Could you check a few things on this model? Use its own coordinates, in mm. A direction names the side the tool comes from. Give positions to 0.01 mm unless a question says otherwise; leave off trailing zeros. Loops run counter-clockwise (first coordinate to the right, second up) from the corner with the lowest first, then second, coordinate; pieces in that order, holes last. Notation, with made-up numbers: (-3, 57) - (13, 57) arc R21 ccw to (13, 74) - close; hole circle Ø7 at (51, 69). An arc over 180 degrees is marked (long way). Use CSV: the item, a comma, the result in double quotes.
from build123d import *

# Parameters (mm, degrees)
ESQUISSE1_W             = 12
ESQUISSE1_H             = 108
ESQUISSE1_R             = 1.6
BOSS_EXTRU_1_DEPTH      = 4
ESQUISSE2_R             = 2.2
BOSS_EXTRU_2_DEPTH      = 4
BOSS_EXTRU_3_DEPTH      = 12
ESQUISSE4_W             = 12
ESQUISSE4_H             = 16
ESQUISSE4_R             = 2.2
BOSS_EXTRU_4_DEPTH      = 6
ENL_V_MAT_EXTRU_1_DEPTH = 13
ESQUISSE6_R             = 4.5
ENL_V_MAT_EXTRU_2_DEPTH = 14
ESQUISSE8_R             = 4.5
ENL_V_MAT_EXTRU_3_DEPTH = 4
ESQUISSE9_R             = 1.6
ENL_V_MAT_EXTRU_4_DEPTH = 17
ESQUISSE10_R            = 3.5
ENL_V_MAT_EXTRU_5_DEPTH = 14
CONG_1_R                = 4
CONG_2_R                = 4
CONG_3_R                = 4


with BuildPart() as part:
    # Esquisse1 → Boss.-Extru.1 (new body)
    with BuildSketch(Plane.XY):
        with Locations((-47.5, 54)):
            Rectangle(ESQUISSE1_W, ESQUISSE1_H)
        with Locations((-47.5, 100)):
            Circle(ESQUISSE1_R, mode=Mode.SUBTRACT)
    extrude(amount=BOSS_EXTRU_1_DEPTH)

    # Esquisse2 → Boss.-Extru.2 (add)
    with BuildSketch(Plane.XZ):
        Polygon((-41.5, 0), (-29.5, 0), (-29.5, 16), (-53.5, 16), (-53.5, 4), (-41.5, 4), align=None)
        with Locations((-37.5, 8)):
            Circle(ESQUISSE2_R, mode=Mode.SUBTRACT)
    extrude(amount=-BOSS_EXTRU_2_DEPTH)

    # Esquisse3 → Boss.-Extru.3 (add)
    with BuildSketch(Plane.ZY.offset(53.5)):
        Polygon((4, 108), (16, 4), (4, 4), align=None)
    extrude(amount=-BOSS_EXTRU_3_DEPTH)

    # Esquisse4 → Boss.-Extru.4 (add)
    with BuildSketch(Plane(origin=(0, 4, 0), x_dir=(1, 0, 0), z_dir=(0, 1, 0))):
        with Locations((-35.5, -8)):
            Rectangle(ESQUISSE4_W, ESQUISSE4_H)
        with Locations((-37.5, -8)):
            Circle(ESQUISSE4_R, mode=Mode.SUBTRACT)
    extrude(amount=BOSS_EXTRU_4_DEPTH)

    # Esquisse5 → Enlèv. mat.-Extru.1 (cut, through all)
    with BuildSketch(Plane.ZY.offset(41.5)):
        Polygon((15.307692308, 10), (16, 4), (16, 10), align=None)
    extrude(amount=-ENL_V_MAT_EXTRU_1_DEPTH, mode=Mode.SUBTRACT)

    # Esquisse6 → Enlèv. mat.-Extru.2 (cut)
    with BuildSketch(Plane(origin=(0, 10, 0), x_dir=(1, 0, 0), z_dir=(0, 1, 0))):
        with Locations((-37.5, -8)):
            Circle(ESQUISSE6_R)
    extrude(amount=ENL_V_MAT_EXTRU_2_DEPTH, mode=Mode.SUBTRACT)

    # Esquisse8 → Enlèv. mat.-Extru.3 (cut)
    with BuildSketch(Plane(origin=(0, 10, 0), x_dir=(1, 0, 0), z_dir=(0, 1, 0))):
        with Locations((-37.5, -8)):
            Circle(ESQUISSE8_R)
    extrude(amount=-ENL_V_MAT_EXTRU_3_DEPTH, mode=Mode.SUBTRACT)

    # Esquisse9 → Enlèv. mat.-Extru.4 (cut, through all)
    with BuildSketch(Plane(origin=(0, 0, 0), x_dir=(-1, 0, 0), z_dir=(0, 0, -1))):
        with Locations((47.5, 100)):
            Circle(ESQUISSE9_R)
    extrude(amount=-ENL_V_MAT_EXTRU_4_DEPTH, mode=Mode.SUBTRACT)

    # Esquisse10 → Enlèv. mat.-Extru.5 (cut, through all)
    with BuildSketch(Plane(origin=(0, 0, 3), x_dir=(-1, 0, 0), z_dir=(0, 0, -1))):
        with Locations((47.5, 100)):
            Circle(ESQUISSE10_R)
    extrude(amount=-ENL_V_MAT_EXTRU_5_DEPTH, mode=Mode.SUBTRACT)

    # Congé1
    cong_1_edges = [part.edges().sort_by_distance(p)[0] for p in [
        (-41.5, 108, 2),
        (-53.5, 108, 2),
    ]]
    fillet(cong_1_edges, radius=CONG_1_R)

    # Congé2
    cong_2_edges = [part.edges().sort_by_distance(p)[0] for p in [
        (-41.5, 10, 2.969223594),
        (-41.5, 10, 12.68462256),
    ]]
    fillet(cong_2_edges, radius=CONG_2_R)

    # Congé3
    cong_3_edges = [part.edges().sort_by_distance(p)[0] for p in [
        (-29.5, 5, 0),
        (-29.5, 7, 15.653846154),
    ]]
    fillet(cong_3_edges, radius=CONG_3_R)


solid = part.part
1) Suppose I cut it at D-D (y = 17.5). Please give me the cut outline in (x, z), plus the area to 3 significant figures.
Answer below:
outline,"(-53.5, 0) - (-41.5, 0) - (-41.5, 5.94) arc R4.5 cw to (-41.5, 10.06) - (-41.5, 14.44) - (-53.5, 14.44) - close"
area,"172 mm2"
2) Suppose I cut it at B-B (y = 100). Please give me the cut outline in (x, z).
Answer below:
outline,"(-53.5, 0) - (-49.1, 0) - (-49.1, 3) - (-51, 3) - (-51, 4.92) - (-53.5, 4.92) - close; (-45.9, 0) - (-41.5, 0) - (-41.5, 4.92) - (-44, 4.92) - (-44, 3) - (-45.9, 3) - close"
3) I'm going to push flat-ended pins straight in: P1, Ø4.5, axis at y = 80, z = 7, coming from the +X side; P2, Ø5.5, axis at x = -47.5, y = 100, coming from the +Z side; P3, Ø2.5, axis at x = -32, z = 7.5, coming from the +Y side; P4, Ø1.9, axis at x = -47.5, y = 100, coming from the +Z side. Where does each tip first touch, or does it pass through?
Answer below:
P1,"stops at x = -41.5"
P2,"stops at z = 3"
P3,"stops at y = 10"
P4,"passes through"
4) Which directions (+Z, -Z, +X, -X, +Y, -Y) give clear straight access to the entire face, cutting with the end or side of a thin tool? Please do faces 5 (the cylindrical face through (-42, 11, 8)), 6 (the flat face through (-41.5, 50, 6)), 7 (the cylindrical face through (-46.741, 96.583, 3.92)).
Answer below:
face 5,"none"
face 6,"+Z, -Z, +X, +Y"
face 7,"+Z"
5) We'd pull the mould along Z, two halves only. Please class faces 1 (the cylindrical face through (-31, 5, 15)), 2 (the cylindrical face through (-30.703, 4.93, 1.141)), 3 (the cylindrical face through (-39.698, 2.958, 8.097)), 4 (the flat face through (-48, 108, 2)): +Z half, -Z half, draft (parallel to the pull), parting line (faces both ways), or undercut.
Answer below:
face 1,"+Z half"
face 2,"-Z half"
face 3,"undercut"
face 4,"draft"
6) Suppose I cut it at A-A (x = -47.5). Please give me the cut outline in (y, z).
Answer below:
outline,"(0, 0) - (98.4, 0) - (98.4, 3) - (96.5, 3) - (96.5, 5.33) - (4, 16) - (0, 16) - close; (101.6, 0) - (108, 0) - (108, 4) - (103.5, 4.52) - (103.5, 3) - (101.6, 3) - close"
7) I need wall thicknesses on line 1 along Z through (x, y) = (-37.5, 1.35); line 2 along X through (y, z) = (100, 1.4); line 3 along Y through (x, z) = (-47.5, 3.7). Which ranges of each line are inside material? Lowest first, please.
Answer below:
line 1,"z = 0 to 5.8, 10.2 to 16"
line 2,"x = -53.5 to -49.1, -45.9 to -41.5"
line 3,"y = 0 to 96.5, 103.5 to 108"
8) Suppose I cut it at C-C (z = 8). Please give me the cut outline in (x, y), plus the area to 3 significant figures.
Answer below:
outline,"(-53.5, 0) - (-39.7, 0) - (-39.7, 6) - (-42, 6) - (-42, 24) - (-41.5, 24) - (-41.5, 73.33) - (-53.5, 73.33) - close; (-35.3, 0) - (-29.5, 0) - (-29.5, 10) - (-33, 10) - (-33, 6) - (-35.3, 6) - close"
area,"931 mm2"
